Model file for the job. Use its own axes, mm. A direction names the side the tool comes from. Give positions to 0.01 mm unless a question says otherwise; leave off trailing zeros. Loops run counter-clockwise (first coordinate to the right, second up) from the corner with the lowest first, then second, coordinate; pieces in that order, holes last. Notation, with made-up numbers: (-38, 12) -> (-16, 12) arc R11 ccw to (-16, 16) -> close; hole circle Ø5 at (62.5, 54). An arc over 180 degrees is marked (long way). Use CSV: the item, a comma, the result in double quotes. Start each with the question number.
(1) Cut at C-C on z = 4.25. Write the cut outline in (x, y), then the cut area to 3 significant figures.
(2) Pull direction X, two halves, no side cores. Call faces 4 (the flat face through (0, 0, 8)), 5 (the cylindrical face through (-0.867, 3.905, 14.79)), 6 (the flat face through (-2, -1, 0)): pulls with the +X half, pulls with the -X half, needs draft (parallel to the pull), parting line crosses it, or undercut.
(3) Cut at A-A on x = 0. Write the cut outline in (y, z), then the cut area to 3 significant figures.
(4) Cut at D-D on z = 14.25. Write the cut outline in (x, y).
(5) Drill centre lines: probe 1 along Y at (x, z) = (0, 2.25); probe 2 along Y at (x, z) = (0.5, 6); probe 3 along Z at (x, y) = (-1, -0.5). Where is each one in solid material? Low to high.
(6) Flat gauge pins, fed straight in: pin 1 (2 mm diameter, centred on x = 0.5, y = 1, fed in from +Z); pin 2 (2.5 mm diameter, centred on x = 0, y = 0, fed in from -Z). Where does each tip first touch, or does it go through?
(7) 3-axis set-ups, long thin cutter, end or side, ignore diameter. For faces 1 (the flat face through (0, 0, 22)), 2 (the cylindrical face through (0, -2, 4)), 3 (the flat face through (-2, -1, 30)): which of +Z, -Z, +X, -X, +Y, -Y reach the whole face in a straight line?
Autodesk Inventor part; units mm, degrees
ref_plane "YZ Plane" through (0, 0, 0) normal (1, 0, 0) x (0, 1, 0)
ref_plane "XZ Plane" through (0, 0, 0) normal (0, 1, 0) x (-1, 0, 0)
ref_plane "XY Plane" through (0, 0, 0) normal (0, 0, 1) x (1, 0, 0)
sketch "スケッチ1" plane through (0, 0, 0) normal (0, 0, 1) x (1, 0, 0)
  circle A0 centre (0, 0) radius 4
  circle A1 centre (0, 0) radius 2
  dimension "d0" = 8
  dimension "d1" = 4
extrude "押し出し1" add sketch "スケッチ1" along normal blind 30 contours A0 | A1
sketch "スケッチ2" plane through (0, 0, 30) normal (0, 0, 1) x (1, 0, 0)
  circle A0 centre (0, 0) radius 2
  dimension "d4" = 4
extrude "押し出し2" cut sketch "スケッチ2" against normal blind 8
sketch "スケッチ3" plane through (0, 0, 0) normal (0, 0, -1) x (-1, 0, 0)
  circle A0 centre (0, 0) radius 2
  dimension "d7" = 4
extrude "押し出し3" cut sketch "スケッチ3" against normal blind 8
properties part number "スペーサーm4,30" material "アルミニウム 7075"
Check result:
1,outline,"circle Ø8 at (0, 0); hole circle Ø4 at (0, 0)"
1,area,"37.7 mm²"
2,face 4,"undercut"
2,face 5,"parting line crosses it"
2,face 6,"needs draft"
3,outline,"(-4, 0) -> (-2, 0) -> (-2, 8) -> (2, 8) -> (2, 0) -> (4, 0) -> (4, 30) -> (2, 30) -> (2, 22) -> (-2, 22) -> (-2, 30) -> (-4, 30) -> close"
3,area,"176 mm²"
4,outline,"circle Ø8 at (0, 0)"
5,probe 1,"-4 to -2, 2 to 4"
5,probe 2,"-3.97 to -1.94, 1.94 to 3.97"
5,probe 3,"8 to 22"
6,pin 1,"z = 30"
6,pin 2,"z = 8"
7,face 1,"+Z"
7,face 2,"-Z"
7,face 3,"+Z, +X, -X, +Y, -Y"
